Here's how the part is built. I have some questions about the finished solid (model axes, mm). A direction names the side the tool comes from. Round coordinates to 2 decimals unless told otherwise and drop trailing zeros. Order: outer loops, then holes, each group sorted by start corner. A loop starts at its lowest first (then second) coordinate and runs counter-clockwise, first axis right, second up. Notation, with made-up numbers: (-12, 71) -> (34, 71) arc R23 ccw to (34, 102) -> close; hole circle Ø3 at (-31.5, 16). An arc over 180 degrees is marked (long way). Answer in a Markdown table with one row per item.
```python
from build123d import *

# Parameters (mm, degrees)
F0_W      = 70
F0_H      = 80
F1_DEPTH  = 5
F2_W      = 2
F2_H      = 42.3
F3_DEPTH  = 42.3
F4_R      = 1.65
F4_R_2    = 10.5
F5_DEPTH  = 25
F7_DEPTH  = 4
F9_DEPTH  = 4
F10_W     = 70
F10_H     = 29.7
F11_DEPTH = 42.3
F12_W     = 42.3
F12_H     = 2
F13_DEPTH = 42.3
F14_R     = 1.65
F14_R_2   = 10.5
F15_DEPTH = 25
F17_DEPTH = 4
F19_DEPTH = 88.9
F21_DEPTH = 4
F22_W     = 19.7
F22_H     = 29.7
F23_DEPTH = 64.9
F24_W     = 53
F24_H     = 2
F25_DEPTH = 45.92
F26_W     = 50.3
F26_H     = 4.7
F27_DEPTH = 73.2
F28_W     = 12
F28_H     = 83
F29_DEPTH = 5
F30_W     = 12
F30_H     = 40
F31_DEPTH = 23
F32_R     = 4.85
F33_DEPTH = 45.2
F35_DEPTH = 25


with BuildPart() as f1:
    # F0 (on Top) → F1 (new body)
    with BuildSketch(Plane.XY):
        with Locations((35, 40)):
            Rectangle(F0_W, F0_H)
    extrude(amount=F1_DEPTH)

    # F2 (on face) → F3 (join)
    with BuildSketch(Plane.XY.offset(5)):
        with Locations((16, 25.15)):
            Rectangle(F2_W, F2_H)
    extrude(amount=F3_DEPTH)

    # F4 (on face) → F5 (cut)
    with BuildSketch(Plane(origin=(15, 0, 0), x_dir=(0, -1, 0), z_dir=(-1, 0, 0))):
        with Locations((-40.65, 41.65)):
            Circle(F4_R)
        with Locations((-9.65, 41.65)):
            Circle(F4_R)
        with Locations((-9.65, 10.65)):
            Circle(F4_R)
        with Locations((-40.65, 10.65)):
            Circle(F4_R)
        with Locations((-25.15, 26.15)):
            Circle(F4_R_2)
    extrude(amount=-F5_DEPTH, mode=Mode.SUBTRACT)

    # F6 (on face) → F7 (join)
    with BuildSketch(Plane(origin=(0, 46.3, 0), x_dir=(-1, 0, 0), z_dir=(0, 1, 0))):
        Polygon((-17, 5), (0, 5), (-15, 47.3), (-17, 47.3), align=None)
    extrude(amount=F7_DEPTH)

    # F8 (on face) → F9 (join)
    with BuildSketch(Plane.XZ.offset(-4)):
        Polygon((17, 5), (17, 47.3), (15, 47.3), (0, 5), (15, 5), align=None)
    extrude(amount=F9_DEPTH)

    # F10 (on face) → F11 (join)
    with BuildSketch(Plane.XY.offset(5)):
        with Locations((35, 65.15)):
            Rectangle(F10_W, F10_H)
    extrude(amount=F11_DEPTH)

    # F12 (on face) → F13 (join)
    with BuildSketch(Plane.XY.offset(47.3)):
        with Locations((44.85, 51.3)):
            Rectangle(F12_W, F12_H)
    extrude(amount=F13_DEPTH)

    # F14 (on face) → F15 (cut)
    with BuildSketch(Plane(origin=(0, 52.3, 0), x_dir=(-1, 0, 0), z_dir=(0, 1, 0))):
        with Locations((-60.35, 83.95)):
            Circle(F14_R)
        with Locations((-29.35, 83.95)):
            Circle(F14_R)
        with Locations((-29.35, 52.95)):
            Circle(F14_R)
        with Locations((-60.35, 52.95)):
            Circle(F14_R)
        with Locations((-44.85, 68.45)):
            Circle(F14_R_2)
    extrude(amount=-F15_DEPTH, mode=Mode.SUBTRACT)

    # F16 (on face) → F17 (join)
    with BuildSketch(Plane.YZ.offset(66)):
        Polygon((52.3, 89.6), (50.3, 89.6), (50.3, 47.3), (75.3, 47.3), align=None)
    extrude(amount=F17_DEPTH)

    # F18 (on face) → F19 (cut)
    with BuildSketch(Plane.XZ.offset(-50.3)):
        Polygon((0, 5), (15, 47.3), (0, 47.3), align=None)
    extrude(amount=-F19_DEPTH, mode=Mode.SUBTRACT)

    # F20 (on face) → F21 (join)
    with BuildSketch(Plane(origin=(23.7, 0, 0), x_dir=(0, -1, 0), z_dir=(-1, 0, 0))):
        Polygon((-50.3, 47.3), (-50.3, 89.6), (-52.3, 89.6), (-75.3, 47.3), align=None)
    extrude(amount=F21_DEPTH)

    # F22 (on face) → F23 (cut)
    with BuildSketch(Plane.XY.offset(47.3)):
        with Locations((9.85, 65.15)):
            Rectangle(F22_W, F22_H)
    extrude(amount=-F23_DEPTH, mode=Mode.SUBTRACT)

    # F24 (on face) → F25 (join)
    with BuildSketch(Plane.XY.offset(47.3)):
        with Locations((43.5, 49.3)):
            Rectangle(F24_W, F24_H)
    extrude(amount=-F25_DEPTH)

    # F26 (on face) → F27 (cut)
    with BuildSketch(Plane.XY.offset(47.3)):
        with Locations((44.85, 77.65)):
            Rectangle(F26_W, F26_H)
    extrude(amount=-F27_DEPTH, mode=Mode.SUBTRACT)

    # F28 (on face) → F29 (join)
    with BuildSketch(Plane.XY.offset(5)):
        with Locations((44.85, -41.5)):
            Rectangle(F28_W, F28_H)
    extrude(amount=-F29_DEPTH)

    # F30 (on face) → F31 (join)
    with BuildSketch(Plane.XY.offset(5)):
        with Locations((44.85, -63)):
            Rectangle(F30_W, F30_H)
    extrude(amount=F31_DEPTH)

    # F32 (on face) → F33 (cut)
    with BuildSketch(Plane.XZ.offset(83)):
        with Locations((44.85, 26.15)):
            Circle(F32_R)
    extrude(amount=-F33_DEPTH, mode=Mode.SUBTRACT)

    # F34 (on face) → F35 (cut)
    with BuildSketch(Plane.XY.offset(5)):
        Polygon((40.5, 24.15), (21, 44.3), (21, 4), align=None)
        Polygon((66, 4), (66, 44.3), (46.5, 24.15), align=None)
        Polygon((62, 44.3), (25, 44.3), (43.5, 26.396774), align=None)
        Polygon((62, 4), (43.5, 21.903226), (25, 4), align=None)
    extrude(amount=-F35_DEPTH, mode=Mode.SUBTRACT)


solid = f1.part
```
1. We'd pull the mould along X, two halves only. Please class faces 1 (the face through (34.38, 13.08, 2.54)), 2 (the face through (11, 4, 17)), 3 (the face through (43, 4, 3)), 4 (the face through (15, 20, 16)): released by +X, released by -X, zero draft, split by the parting line, or undercut.
Numbers:
| item | result |
|---|---|
| face 1 | undercut |
| face 2 | zero draft |
| face 3 | undercut |
| face 4 | released by -X |
2. Suppose I cut it at D-D on x = 29.35. State how many separate pieces and enclosed holes the cut face has, then the cut area to 3 significant figures.
Numbers:
| item | result |
|---|---|
| separate pieces | 6 |
| enclosed holes | 0 |
| area | 1,430 mm2 |
3. For faces 5 (the face through (43, 3, 5)), 6 (the face through (45, 64, 47.3)), 7 (the face through (7, 25, 5)), 8 (the face through (56.39, 34.37, 2.54)), which set-ups out of +Z, -Z, +X, -X, +Y, -Y let a thin tool reach every point of the face, with its end or its side?
Numbers:
| item | result |
|---|---|
| face 5 | +Z, +X |
| face 6 | +Z, +Y |
| face 7 | +Z, -X |
| face 8 | +Z, -Z |
4. Suppose I cut it at A-A on z = 68.45. Write out the boundary of the cut face in (x, y).
Numbers:
| item | result |
|---|---|
| outline | (19.7, 50.3) -> (34.35, 50.3) -> (34.35, 52.3) -> (23.7, 52.3) -> (23.7, 63.8) -> (19.7, 63.8) -> close; (55.35, 50.3) -> (70, 50.3) -> (70, 63.8) -> (66, 63.8) -> (66, 52.3) -> (55.35, 52.3) -> close |
5. Please list where these lines run through material, in increasing order: line 1 along Z through (x, y) = (16, 25); line 2 along X through (y, z) = (51, 83); line 3 along X through (y, z) = (-69.5, 26.15).
Numbers:
| item | result |
|---|---|
| line 1 | z = 0 to 15.65, 36.65 to 47.3 |
| line 2 | x = 19.7 to 28, 30.7 to 59, 61.7 to 70 |
| line 3 | x = 38.85 to 40, 49.7 to 50.85 |
6. Suppose I cut it at B-B on y = 40.65. Write out the boundary of the cut face in (x, z).
Numbers:
| item | result |
|---|---|
| outline | (0, 0) -> (21, 0) -> (21, 5) -> (17, 5) -> (17, 9) -> (15, 9) -> (15, 5) -> (0, 5) -> close; (15, 12.3) -> (17, 12.3) -> (17, 40) -> (15, 40) -> close; (15, 43.3) -> (17, 43.3) -> (17, 47.3) -> (15, 47.3) -> close; (24.53, 0) -> (28.77, 0) -> (28.77, 5) -> (24.53, 5) -> close; (58.23, 0) -> (62.47, 0) -> (62.47, 5) -> (58.23, 5) -> close; (66, 0) -> (70, 0) -> (70, 5) -> (66, 5) -> close |
7. Suppose I cut it at C-C on x = 52.5. Write out the boundary of the cut face in (y, z).
Numbers:
| item | result |
|---|---|
| outline | (0, 0) -> (4, 0) -> (4, 5) -> (0, 5) -> close; (13.19, 0) -> (17.95, 0) -> (17.95, 5) -> (13.19, 5) -> close; (30.35, 0) -> (35.11, 0) -> (35.11, 5) -> (30.35, 5) -> close; (44.3, 0) -> (75.3, 0) -> (75.3, 47.3) -> (52.3, 47.3) -> (52.3, 61.26) -> (50.3, 61.26) -> (50.3, 47.3) -> (48.3, 47.3) -> (48.3, 5) -> (44.3, 5) -> close; (50.3, 75.64) -> (52.3, 75.64) -> (52.3, 89.6) -> (50.3, 89.6) -> close |
8. For pin 1 Ø12.5 at (y, z) = (17, 24.5) entering from -X; pin 2 Ø5.5 at (y, z) = (9.65, 10.65) entering from +X; pin 3 Ø10 at (x, z) = (37.5, 78) entering from -Y; pin 4 Ø17 at (x, z) = (44.85, 68.45) entering from -Y, each with a flat end and sliding along its axis, tell me the tip position at first contact or that it passes through.
Numbers:
| item | result |
|---|---|
| pin 1 | stops at x = 15 |
| pin 2 | stops at x = 17 |
| pin 3 | stops at y = 50.3 |
| pin 4 | passes through |
